Autodesk Inventor part; units mm, degrees
ref_plane "Plano de trabalho1" through (0, 160, 0) normal (0, 1, 0) x (-1, 0, 0)
ref_plane "Plano de trabalho2" through (0, -175, 0) normal (0, 1, 0) x (-1, 0, 0)
ref_plane "YZ Plane" through (0, 0, 0) normal (1, 0, 0) x (0, 1, 0)
sketch "Esboço1" plane through (0, 0, 0) normal (0, 0, 1) x (1, 0, 0)
  circle A0 centre (0, 0) radius 140
  circle A1 centre (0, 0) radius 96
  dimension "d0" = 280
  dimension "d1" = 192
extrude "Extrusão1" add sketch "Esboço1" along normal mid plane 225
ref_plane "Plano de trabalho1" through (0, 160, 0) normal (0, 1, 0) x (-1, 0, 0)
sketch "Esboço2" plane through (0, 160, 0) normal (0, 1, 0) x (-1, 0, 0)
  circle A0 centre (0, 0) radius 100
  dimension "d5" = 200
extrude "Extrusão2" add sketch "Esboço2" against normal up to next
ref_plane "Plano de trabalho2" through (0, -175, 0) normal (0, 1, 0) x (-1, 0, 0)
sketch "Esboço3" plane through (0, -175, 0) normal (0, 1, 0) x (-1, 0, 0)
  circle A0 centre (0, 0) radius 37.5
  dimension "d9" = 75
extrude "Extrusão3" add sketch "Esboço3" along normal up to next
sketch "Esboço4" plane through (0, 160, 0) normal (0, 1, 0) x (1, 0, 0)
  circle A0 centre (0, 0) radius 50
  dimension "d12" = 100
extrude "Extrusão4" cut sketch "Esboço4" against normal blind 25
sketch "Esboço5" plane through (0, 135, 0) normal (0, 1, 0) x (1, 0, 0)
  circle A0 centre (0, 0) radius 28
  dimension "d15" = 56
extrude "Extrusão5" cut sketch "Esboço5" against normal blind 285
sketch "Esboço6" plane through (0, 160, 0) normal (0, 1, 0) x (1, 0, 0)
  circle A0 centre (0, 75) radius 10
  circle A1 centre (-64.9519, -37.5) radius 10
  circle A2 centre (64.9519, -37.5) radius 10
  point P0 (0, 0)
  dimension "d18" = 20
  dimension "d19" = 75
  dimension "d22" = 360
extrude "Extrusão6" cut sketch "Esboço6" against normal blind 15
sketch "Esboço7" plane through (0, 0, 112.5) normal (0, 0, 1) x (1, 0, 0)
  arc A0 (-50, -185) -> (50, -185) centre (0, -185) ccw
  circle A1 centre (0, -185) radius 23.5
  line L0 (50, -185) -> (50, -106.8082)
  line L1 (-50, -185) -> (-50, -106.8082)
  line L2 (50, -106.8082) -> (-50, -106.8082)
  point P0 (0, 0)
  dimension "d26" = 100
  dimension "d27" = 47
  dimension "d28" = 185
extrude "Extrusão7" add sketch "Esboço7" against normal blind 32
pattern_circular "Padrão circular1" count 3 over 360 about axis through (0, 0, 0) along (0, 0, 1) of "Extrusão7"
mirror "Espelhamento1" about plane through (0, 0, 0) normal (0, 0, 1) of "Extrusão7", "Padrão circular1"
properties part number "Corpo da Valvula"
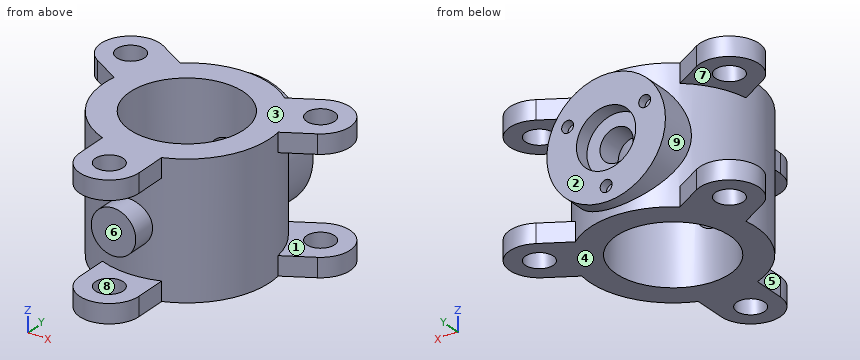
Geometry: final body of the model. Coordinates: model frame, mm. Face numbers are marked on the shaded views. A direction names the side the tool comes from. Give positions to 0.01 mm unless a question says otherwise; leave off trailing zeros. Write each loop counter-clockwise with the first axis right and the second up, starting at its lowest first coordinate (ties: lowest second). Pieces come first, ordered by that corner, then holes. Notation, with made-up numbers: M 46.25,46.5 L 69.25,46.5 A9 cw 69.25,54.5 Z; hole C 62.25,66 d6. An arc over 180 degrees is marked long. Answer in a Markdown table with one row per item. Add a question column.
(1) Ray query, line 1 (Z direction, x = 0, y = 142.5); line 2 (Z direction, x = 0, y = 104); line 3 (X direction, y = 149, z = 37.5). Return the intervals inside material, ascending.
(2) Mould query, pull axis Z, two halves, no side actions, for the marked faces 1, 2, 3 and 4. Classes: +Z half, -Z half, draft (parallel to the pull), parting line (faces both ways), or undercut.
(3) Section C-C on x = 0. State how many separate pieces and enclosed holes the cut face has, and give its area (3 significant figures).
(4) First-contact query: pin 1 (22 mm diameter, centred on x = 61.5, z = 34, fed in from +Y); pin 2 (6 mm diameter, centred on x = 1, z = -79.5, fed in from +Y); pin 3 (1 mm diameter, centred on x = 102.5, z = -63, fed in from -Y); pin 4 (9.5 mm diameter, centred on y = -149, z = 89.5, fed in from +X). Flat tips, straight axial feed; report the tip coordinate or a pass-through.
(5) Section B-B on z = -75. Return loops of the section in (x, y), and give its area (3 significant figures).
(6) Reachability of the marked faces 5, 6, 7, 8 and 9 from +Z, -Z, +X, -X, +Y, -Y: full face, straight path, thin tool, end or side. Return the list, or none.
(7) Section A-A on y = 0. Return loops of the section in (x, z).
(8) Section D-D on z = 0. Return loops of the section in (x, y), and give its area (3 significant figures).
Result set:
| question | item | result |
|---|---|---|
| 1 | line 1 | z = -100 to -50, 50 to 100 |
| 1 | line 2 | z = -112.5 to -28, 28 to 112.5 |
| 1 | line 3 | x = -92.7 to -74.95, -54.95 to -33.07, 33.07 to 54.95, 74.95 to 92.7 |
| 2 | face 1 | undercut |
| 2 | face 2 | draft |
| 2 | face 3 | +Z half |
| 2 | face 4 | -Z half |
| 3 | separate pieces | 5 |
| 3 | enclosed holes | 0 |
| 3 | area | 21,500 mm^2 |
| 4 | pin 1 | stops at y = 160 |
| 4 | pin 2 | stops at y = 145 |
| 4 | pin 3 | stops at y = -95.9 |
| 4 | pin 4 | stops at x = 50 |
| 5 | outline | M -66.14,123.39 A140 ccw long 66.14,123.39 L 66.14,160 L 10,160 L 10,145 L -10,145 L -10,160 L -66.14,160 Z; hole C 0,0 d192 |
| 5 | area | 35,700 mm^2 |
| 6 | face 5 | +Z, -Z, -X, -Y |
| 6 | face 6 | +X, -X, -Y |
| 6 | face 7 | -X, +Y |
| 6 | face 8 | -Z |
| 6 | face 9 | +Y |
| 7 | outline | M -140,-112.5 L -96,-112.5 L -96,112.5 L -140,112.5 Z; M 96,-112.5 L 140,-112.5 L 140,112.5 L 96,112.5 Z |
| 8 | outline | M -100,97.98 A140 ccw -37.5,-134.88 L -37.5,-175 L 37.5,-175 L 37.5,-134.88 A140 ccw 100,97.98 L 100,160 L 50,160 L 50,135 L 28,135 L 28,91.83 A96 cw 28,-91.83 L 28,-150 L -28,-150 L -28,-91.83 A96 cw -28,91.83 L -28,135 L -50,135 L -50,160 L -100,160 Z |
| 8 | area | 34,100 mm^2 |
